from build123d import *

# Parameters (mm, degrees)
F0_W     = 66.04
F0_H     = 10.16
F1_DEPTH = 12.7
F2_W     = 12.7
F2_H     = 12.7
F3_DEPTH = 5.08
F2_W_2   = 5.08
F4_DEPTH = 2.54


with BuildPart() as f1:
    # F0 (on Top) → F1 (new body)
    with BuildSketch(Plane.XY):
        with Locations((33.02, -5.08)):
            Rectangle(F0_W, F0_H)
    extrude(amount=F1_DEPTH)

    # F2 (on face) → F3 (join)
    with BuildSketch(Plane(origin=(0, 0, 0), x_dir=(-1, 0, 0), z_dir=(0, 1, 0))):
        with Locations((-24.13, 6.35)):
            Rectangle(F2_W, F2_H)
        with Locations((-41.91, 6.35)):
            Rectangle(F2_W, F2_H)
    extrude(amount=F3_DEPTH)

    # F2 (on face) → F4 (join)
    with BuildSketch(Plane(origin=(0, 0, 0), x_dir=(-1, 0, 0), z_dir=(0, 1, 0))):
        with Locations((-15.24, 6.35)):
            Rectangle(F2_W_2, F2_H)
        with Locations((-33.02, 6.35)):
            Rectangle(F2_W_2, F2_H)
        with Locations((-50.8, 6.35)):
            Rectangle(F2_W_2, F2_H)
    extrude(amount=F4_DEPTH)


solid = f1.part
The listing builds one solid part. Answer for the finished solid, in the listing's coordinates (mm). A direction names the side the tool comes from. Round coordinates to 2 decimals unless told otherwise and drop trailing zeros. Order: outer loops, then holes, each group sorted by start corner. A loop starts at its lowest first (then second) coordinate and runs counter-clockwise, first axis right, second up. Notation, with made-up numbers: M -21,51.25 L 23,51.25 A31 cw 23,82.25 Z; hole C 39.5,-20 d10. An arc over 180 degrees is marked long. Answer in a Markdown table with one row per item. Add a question column.
1) Determine the mould class of faces 1 (the face through (33, 2.54, 6)), 2 (the face through (33, -4, 0)), 3 (the face through (0, -5, 6)) for opening direction X: pulls with the +X half, pulls with the -X half, needs draft (parallel to the pull), parting line crosses it, or undercut.
2) The part is cut by section B-B on x = 33.5. Determine the outline of the cut face in (y, z).
3) Which of the six approach directions +Z, -Z, +X, -X, +Y, -Y give full straight-line access (tool end or side, diameter ignored) to faces 4 (the face through (51, 2.54, 6)), 5 (the face through (42, 5.08, 6)), 6 (the face through (35.56, 4, 6)), 7 (the face through (6, 0, 6))?
4) The part is cut by section A-A on z = 9. Determine the outline of the cut face in (x, y), plus the area to 3 significant figures.
5) Consider line 1 along X through (y, z) = (4, 8); line 2 along Y through (x, z) = (9, 4); line 3 along X through (y, z) = (2, 6.75). Determine where each line is inside the solid, lowest interval first. Write a range as from..to.
6) Flat-ended cylindrical pins translate along their axes: pin 1 Ø3 at (y, z) = (3.5, 3.5) entering from -X; pin 2 Ø0.8 at (y, z) = (3.5, 3.5) entering from +X; pin 3 Ø2.5 at (x, z) = (50, 6.5) entering from +Y. Find the tip coordinate at first contact, or state that the pin passes through.
7) The part is cut by section C-C on y = 1.5. Determine the outline of the cut face in (x, z).
Findings below:
| question | item | result |
|---|---|---|
| 1 | face 1 | undercut |
| 1 | face 2 | needs draft |
| 1 | face 3 | pulls with the -X half |
| 2 | outline | M -10.16,0 L 2.54,0 L 2.54,12.7 L -10.16,12.7 Z |
| 3 | face 4 | +Z, -Z, +X, +Y |
| 3 | face 5 | +Z, -Z, +X, -X, +Y |
| 3 | face 6 | +Z, -Z, +Y |
| 3 | face 7 | +Z, -Z, -X, +Y |
| 4 | outline | M 0,-10.16 L 66.04,-10.16 L 66.04,0 L 53.34,0 L 53.34,2.54 L 48.26,2.54 L 48.26,5.08 L 35.56,5.08 L 35.56,2.54 L 30.48,2.54 L 30.48,5.08 L 17.78,5.08 L 17.78,2.54 L 12.7,2.54 L 12.7,0 L 0,0 Z |
| 4 | area | 839 mm² |
| 5 | line 1 | x = 17.78..30.48, 35.56..48.26 |
| 5 | line 2 | y = -10.16..0 |
| 5 | line 3 | x = 12.7..53.34 |
| 6 | pin 1 | stops at x = 12.7 |
| 6 | pin 2 | stops at x = 48.26 |
| 6 | pin 3 | stops at y = 2.54 |
| 7 | outline | M 12.7,0 L 53.34,0 L 53.34,12.7 L 12.7,12.7 Z |
